Source: CAD feature listing. Evaluate the final solid. Frame: model axes, mm. Round coordinates to 2 decimals unless told otherwise and drop trailing zeros. Order: outer loops, then holes, each group sorted by start corner. A loop starts at its lowest first (then second) coordinate and runs counter-clockwise, first axis right, second up. Notation, with made-up numbers: (45, 21.5) -> (94, 21.5) arc R24 ccw to (94, 53.5) -> close; hole circle Ø2 at (-2, 41.5). An arc over 180 degrees is marked (long way). One line per item, written item: value. Start each with the question number.
1) Section A-A (x = 15). Return the cut outline in (y, z), and give its area (3 significant figures).
2) Pin query (flat end, axial travel): P1, Ø1.2, axis at x = 31, y = 1.5, coming from the -Z side; P2, Ø2, axis at y = 3, z = -16, coming from the +X side; P3, Ø1.2, axis at x = 45, y = 2.5, coming from the +Z side. Return the tip coordinate at first contact, or that it passes through.
3) Section B-B (z = -34.5). Return the cut outline in (x, y).
4) Ray query, L1, parallel to X at y = 0.4, z = -45.5; L2, parallel to Z at x = 44.5, y = 3.3; L3, parallel to X at y = 2.65, z = -14. Return the intervals inside material, ascending.
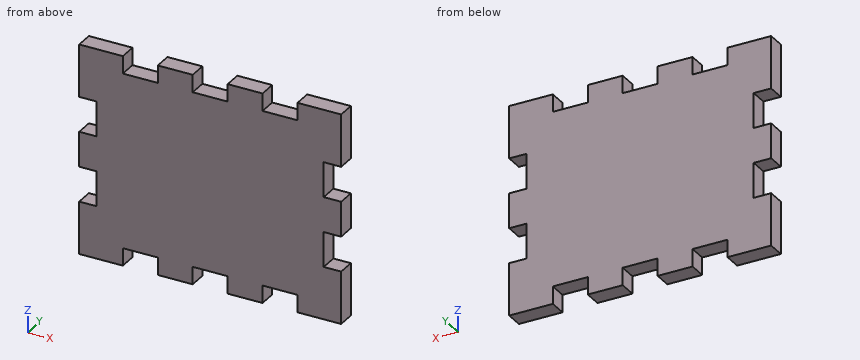
Autodesk Inventor part; units mm, degrees
ref_plane "YZ Plane" through (0, 0, 0) normal (1, 0, 0) x (0, 1, 0)
ref_plane "XZ Plane" through (0, 0, 0) normal (0, 1, 0) x (-1, 0, 0)
ref_plane "XY Plane" through (0, 0, 0) normal (0, 0, 1) x (1, 0, 0)
sketch "Sketch1" plane through (0, 0, 0) normal (0, 1, 0) x (-1, 0, 0)
  line L0 (0, 0) -> (-60, 0)
  line L1 (-60, 0) -> (-60, -48)
  line L2 (-60, -48) -> (0, -48)
  line L3 (0, -48) -> (0, 0)
  dimension "d0" = 60
  dimension "d1" = 48
extrude "Extrusion1" add sketch "Sketch1" along normal blind 4
sketch "Sketch2" plane through (0, 4, 0) normal (0, 1, 0) x (1, 0, 0)
  line L0 (0, 0) -> (60, 0) construction
  line L1 (60, 0) -> (60, 48) construction
  line L2 (60, 48) -> (0, 48) construction
  line L3 (0, 48) -> (0, 0) construction
  line L4 (4, 44) -> (56, 44) construction
  line L5 (56, 44) -> (56, 4) construction
  line L6 (56, 4) -> (4, 4) construction
  line L7 (4, 4) -> (4, 44) construction
  line L8 (60, 48) -> (0, 48) construction
  line L9 (30, 48) -> (30, 0) construction
  line L10 (0, 0) -> (60, 0) construction
  line L11 (0, 48) -> (0, 0) construction
  line L12 (0, 24) -> (60, 24) construction
  line L13 (60, 0) -> (60, 48) construction
  line L14 (0, 28) -> (4, 28)
  line L15 (0, 36) -> (4, 36)
  line L16 (10, 48) -> (10, 44)
  line L17 (10, 44) -> (18, 44)
  line L18 (18, 44) -> (18, 48)
  line L19 (18, 48) -> (10, 48)
  line L20 (26, 48) -> (26, 44)
  line L21 (26, 44) -> (30, 44)
  line L22 (26, 48) -> (30, 48)
  line L23 (0, 36) -> (0, 28)
  line L24 (4, 28) -> (4, 36)
  line L25 (60, 28) -> (56, 28)
  line L26 (60, 36) -> (56, 36)
  line L27 (50, 48) -> (50, 44)
  line L28 (50, 44) -> (42, 44)
  line L29 (42, 44) -> (42, 48)
  line L30 (42, 48) -> (50, 48)
  line L31 (34, 48) -> (34, 44)
  line L32 (34, 44) -> (30, 44)
  line L33 (34, 48) -> (30, 48)
  line L34 (60, 36) -> (60, 28)
  line L35 (56, 28) -> (56, 36)
  line L36 (60, 0) -> (0, 0) construction
  line L37 (4, 4) -> (56, 4) construction
  line L38 (60, 0) -> (0, 0) construction
  line L39 (0, 20) -> (4, 20)
  line L40 (0, 12) -> (4, 12)
  line L41 (10, 0) -> (10, 4)
  line L42 (10, 4) -> (18, 4)
  line L43 (18, 4) -> (18, 0)
  line L44 (18, 0) -> (10, 0)
  line L45 (26, 0) -> (26, 4)
  line L46 (26, 4) -> (30, 4)
  line L47 (26, 0) -> (30, 0)
  line L48 (0, 12) -> (0, 20)
  line L49 (4, 20) -> (4, 12)
  line L50 (34, 0) -> (34, 4)
  line L51 (34, 4) -> (30, 4)
  line L52 (34, 0) -> (30, 0)
  line L53 (42, 4) -> (42, 0)
  line L54 (50, 4) -> (42, 4)
  line L55 (42, 0) -> (50, 0)
  line L56 (50, 0) -> (50, 4)
  line L57 (56, 20) -> (56, 12)
  line L58 (60, 12) -> (56, 12)
  line L59 (60, 12) -> (60, 20)
  line L60 (60, 20) -> (56, 20)
  dimension "d4" = 4
  dimension "d7" = 8
  dimension "d8" = 8
  dimension "d9" = 4
  dimension "d10" = 8
  dimension "d11" = 4
extrude "Extrusion2" cut sketch "Sketch2" against normal up to surface (4 mm away)
properties part number "left" material "PBT Plastic Black"
Findings:
1. outline: (0, -44) -> (4, -44) -> (4, -4) -> (0, -4) -> close
1. area: 160 mm2
2. P1: z = -44
2. P2: x = 56
2. P3: z = -4
3. outline: (4, 0) -> (56, 0) -> (56, 4) -> (4, 4) -> close
4. L1: 0 to 10, 18 to 26, 34 to 42, 50 to 60
4. L2: -44 to -4
4. L3: 4 to 56
